Design review of the part built by this model. Coordinates are the model's own, in mm. Face numbers are marked on the shaded views. A direction names the side the tool comes from. Round coordinates to 2 decimals unless told otherwise and drop trailing zeros. Write each loop counter-clockwise with the first axis right and the second up, starting at its lowest first coordinate (ties: lowest second). Pieces come first, ordered by that corner, then holes. Notation, with made-up numbers: (30.25, -21) - (74.25, -21) arc R24 ccw to (74.25, 18) - close; hole circle Ø11 at (36, 89). An arc over 180 degrees is marked (long way). Use one line per item in the form item = value.
Autodesk Inventor part; units mm, degrees
ref_plane "YZ Plane" through (0, 0, 0) normal (1, 0, 0) x (0, 1, 0)
ref_plane "XZ Plane" through (0, 0, 0) normal (0, 1, 0) x (-1, 0, 0)
ref_plane "XY Plane" through (0, 0, 0) normal (0, 0, 1) x (1, 0, 0)
sketch "Sketch1" plane through (0, 0, 0) normal (1, 0, 0) x (0, 1, 0)
  point P0 (0, 0)
sketch "Sketch2" plane through (0, 0, 0) normal (0, 0, 1) x (1, 0, 0)
  circle A0 centre (0, 0) radius 30.48
  dimension "d0" = 60.96
extrude "Extrusion1" add sketch "Sketch2" along normal blind 116.84
sketch "Sketch3" plane through (0, 0, 116.84) normal (0, 0, 1) x (1, 0, 0)
  line L0 (-39.8452, 52.8156) -> (35.072, 52.8156)
  line L1 (35.072, 52.8156) -> (35.072, 13.178)
  line L2 (35.072, 13.178) -> (-39.8452, 13.178)
  line L3 (-39.8452, 13.178) -> (-39.8452, 52.8156)
  line L4 (-67.2387, 32.9968) -> (-10.3763, 32.9968)
  line L5 (-10.3763, 32.9968) -> (-10.3763, -41.1941)
  line L6 (-10.3763, -41.1941) -> (-67.2387, -41.1941)
  line L7 (-67.2387, -41.1941) -> (-67.2387, 32.9968)
  line L8 (-33.6194, -53.8532) -> (43.5806, -53.8532)
  line L9 (43.5806, -53.8532) -> (43.5806, -7.7823)
  line L10 (43.5806, -7.7823) -> (-33.6194, -7.7823)
  line L11 (-33.6194, -7.7823) -> (-33.6194, -53.8532)
  line L12 (52.9193, 35.3833) -> (13.0742, 35.3833)
  line L13 (13.0742, 35.3833) -> (13.0742, -35.1758)
  line L14 (13.0742, -35.1758) -> (52.9193, -35.1758)
  line L15 (52.9193, -35.1758) -> (52.9193, 35.3833)
  point P0 (0, 0)
  point P1 (-10.3763, 13.178)
  point P2 (13.0742, 13.178)
  point P3 (13.0742, -7.7823)
  point P4 (-10.3763, -7.7823)
  point P5 (-39.8452, 32.9968)
  point P6 (-33.6194, -41.1941)
  point P7 (43.5806, -35.1758)
  point P8 (35.072, 35.3833)
extrude "Extrusion2" cut sketch "Sketch3" against normal blind 20.32 contours L0 L1 L12 L13 L2 L5 L4 L3 | L4 L5 L2 L3 | L3 L2 L5 L10 L11 L6 L7 L4 | L12 L15 L14 L9 L10 L13 L2 L1 | L1 L2 L13 L12 | L10 L13 L14 L9 L8 L11 L6 L5 | L5 L6 L11 L10 | L10 L9 L14 L13
sketch "Sketch4" plane through (0, 0, 116.84) normal (0, 0, 1) x (1, 0, 0)
  point P0 (0, 0)
  point P1 (0.3979, 2.5556)
hole "Hole1" at (0.3979, 2.5556, 116.84) direction (0, 0, -1) diameter 18 end through all
sketch "Sketch5" plane through (0, 0, 0) normal (0, 0, -1) x (-1, 0, 0)
  circle A0 centre (0, 0) radius 24.6156
extrude "Extrusion3" cut sketch "Sketch5" against normal blind 88.9
chamfer "Chamfer1" distance 3.175 angle 45 2 edges at (0.3979, 11.5556, 88.9) (0.3979, 11.5556, 116.84)
chamfer "Chamfer2" distance 5 angle 45 1 edges at (24.6156, 0, 88.9)
sketch "Sketch6" plane through (0, 0, 0) normal (0, 1, 0) x (-1, 0, 0)
  circle A0 centre (0, 27.9124) radius 3.5462
  point P0 (0, 0)
extrude "Extrusion4" cut sketch "Sketch6" against normal blind 88.9
properties part number "storage pipe 2"
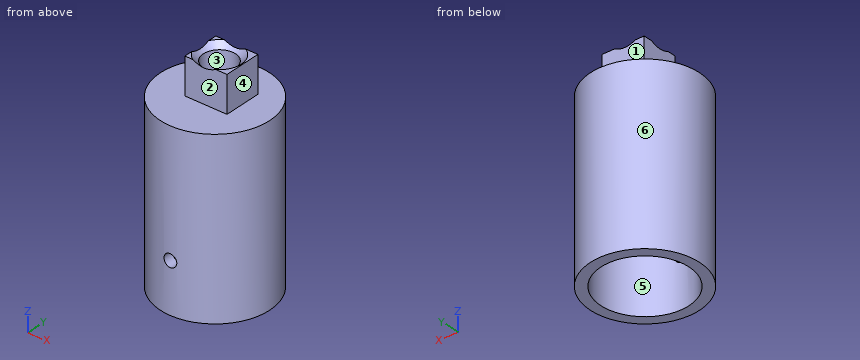
Q1. We need section B-B on x = -1. State how many separate pieces and enclosed holes the cut face has, then the cut area to 3 significant figures.
Calculated:
separate_pieces = 3
enclosed_holes = 0
area = 1,400 mm2
Q2. For P1, Ø4, axis at x = 23, z = 13.5, coming from the -Y side; P2, Ø10, axis at x = 0.5, z = 111.5, coming from the +Y side; P3, Ø5, axis at y = -9, z = 29.5, coming from the -X side, all flat-tipped, find the tip position at first contact; note any pin that passes through.
Calculated:
P1 = -22.09
P2 = 13.18
P3 = -29.78
Q3. Draft analysis for pull direction Y (two halves, no side actions). For the marked faces 1, 2 and 3, state which applies: released by +Y, released by -Y, zero draft, split by the parting line, or undercut.
Calculated:
face_1 = released by +Y
face_2 = released by -Y
face_3 = undercut
Q4. We need section A-A on z = 9.5. Write out the cut boundary in (x, y).
Calculated:
outline = circle Ø60.96 at (0, 0); hole circle Ø49.23 at (0, 0)
Q5. We need section C-C on z = 104.5. Write out the cut boundary in (x, y).
Calculated:
outline = (-10.38, -7.78) - (13.07, -7.78) - (13.07, 13.18) - (-10.38, 13.18) - close; hole circle Ø18 at (0.4, 2.56)
Q6. Machinability: for the marked faces 4, 5 and 6, which of the approach directions +Z, -Z, +X, -X, +Y, -Y give a long, thin tool a straight path to every point of the face, cutting with its end or side? Answer none if there is none.
Calculated:
face_4 = +Z, +X, +Y, -Y
face_5 = -Z
face_6 = +Z, -Z
Q7. To check wall thickness, follow line 1 along Z through (x, y) = (0, -27); line 2 along Y through (x, z) = (-1, 35.5); line 3 along Z through (x, y) = (25.5, 7). State the ranges of each line that lie inside material, in increasing order. Write a range as from..to.
Calculated:
line_1 = 0..24.37, 31.46..96.52
line_2 = -30.46..-24.6, 24.6..30.46
line_3 = 0..96.52
